Geometry: final body of the model. Coordinates: model frame, mm. A direction names the side the tool comes from. Give positions to 0.01 mm unless a question says otherwise; leave off trailing zeros. Order: outer loops, then holes, each group sorted by start corner. A loop starts at its lowest first (then second) coordinate and runs counter-clockwise, first axis right, second up. Notation, with made-up numbers: (8, 64) -> (52, 64) arc R22 cw to (52, 86) -> close; hole circle Ø7 at (34.5, 60.25). An arc over 180 degrees is marked (long way). One line per question, with ' | ' between items. Start each with the question number.
(1) Mould query, pull axis Z, two halves, no side actions, for faces 1 (the face through (1.4, -17.4, -40)), 2 (the face through (-7.66, 5.76, -1.7)), 3 (the face through (13.876, -6.451, -0.56)). Classes: +Z half, -Z half, draft (parallel to the pull), parting line (faces both ways), or undercut.
(2) First-contact query: pin 1 Ø3 at (y, z) = (-14, 29) entering from +X; pin 2 Ø4 at (y, z) = (5.68, 0) entering from -X; pin 3 Ø4 at (x, z) = (13.5, -26.5) entering from +Y. Flat tips, straight axial feed; report the tip coordinate or a pass-through.
(3) Section D-D (z = 0). State how many separate pieces and enclosed holes the cut face has, then the cut area to 3 significant figures.
(4) Set-up query: faces 4 (the face through (-10, 5, -2.85)), 5 (the face through (-13.907, -6.549, -0.56)), 6 (the face through (-10, 5, 4.856)). Return all of +Z, -Z, +X, -X, +Y, -Y with unobstructed straight access to the full face (end or side cutting, diameter ignored); none if empty.
(5) Section A-A (z = -13). Return loops of the section in (x, y), then the cut area to 3 significant figures.
(6) Section C-C (y = -13.5). Return loops of the section in (x, z).
(7) Section B-B (x = 0). Return loops of the section in (y, z), then the cut area to 3 significant figures.
(8) Ray query, L1, parallel to Y at x = -7.2, z = 0; L2, parallel to Y at x = -11.5, z = -14; L3, parallel to Z at x = -9.5, y = 8. Return the intervals inside material, ascending.
```python
from build123d import *

# Parameters (mm, degrees)
EXTRUDE_1_DEPTH     = 40
CUT_EXTRUDE_3_DEPTH = 81
SKETCH_8_R          = 6.65
CUT_EXTRUDE_4_DEPTH = 21
SKETCH_9_R          = 8.65
SKETCH_9_R_2        = 6.65
EXTRUDE_2_DEPTH     = 10
SKETCH_10_W         = 2.6
SKETCH_10_H         = 5.7
EXTRUDE_3_DEPTH     = 10
SKETCH_11_R         = 1.7
CUT_EXTRUDE_5_DEPTH = 10
FILLET_1_R          = 1


with BuildPart() as part:
    # 草图1 → 凸台-拉伸1 (new body, symmetric)
    with BuildSketch(Plane.XY):
        Polygon((-15, 0), (15, 0), (18.130448736, -10), (15, -20), (-15, -20), (-18.130448736, -10), align=None)
    extrude(amount=EXTRUDE_1_DEPTH, both=True)

    # 草图7 → 切除-拉伸3 (cut, through all)
    with BuildSketch(Plane(origin=(0, 0, -40), x_dir=(-1, 0, 0), z_dir=(0, 0, -1))):
        Polygon((14.986888042, -10), (12.795573927, -3), (-12.795573927, -3), (-14.986888042, -10), (-12.795573927, -17), (12.795573927, -17), align=None)
    extrude(amount=-CUT_EXTRUDE_3_DEPTH, mode=Mode.SUBTRACT)

    # 草图8 → 切除-拉伸4 (cut, through all)
    with BuildSketch(Plane(origin=(0, 0, 0), x_dir=(1, 0, 0), z_dir=(0, 1, 0))):
        Circle(SKETCH_8_R)
    extrude(amount=-CUT_EXTRUDE_4_DEPTH, mode=Mode.SUBTRACT)

    # 草图9 → 凸台-拉伸2 (add)
    with BuildSketch(Plane(origin=(0, 0, 0), x_dir=(1, 0, 0), z_dir=(0, 1, 0))):
        Circle(SKETCH_9_R)
        Circle(SKETCH_9_R_2, mode=Mode.SUBTRACT)
    extrude(amount=EXTRUDE_2_DEPTH)

    # 草图10 → 凸台-拉伸3 (add)
    with BuildSketch(Plane(origin=(0, 0, 0), x_dir=(1, 0, 0), z_dir=(0, 1, 0))):
        with BuildLine():
            ThreePointArc((-7.158670401, -4.855505955), (-8.65, 0), (-7.158670401, 4.855505955))
            Line((-7.158670401, 4.855505955), (-13.461589548, 4.855505955))
            Line((-13.461589548, 4.855505955), (-13.461589548, -4.855505955))
            Line((-13.461589548, -4.855505955), (-7.158670401, -4.855505955))
        make_face()
        with Locations((-10.161589548, 0)):
            Rectangle(SKETCH_10_W, SKETCH_10_H, mode=Mode.SUBTRACT)
    extrude(amount=EXTRUDE_3_DEPTH)

    # 草图11 → 切除-拉伸5 (cut)
    with BuildSketch(Plane.ZY.offset(13.461589548)):
        with Locations((0, 5.684678401)):
            Circle(SKETCH_11_R)
    extrude(amount=-CUT_EXTRUDE_5_DEPTH, mode=Mode.SUBTRACT)

    # 圆角1
    fillet_1_edges = [part.edges().sort_by_distance(p)[0] for p in [
        (-13.461589548, 5, -4.855505955),
        (-13.461589548, 5, 4.855505955),
        (-7.158670401, 5, 4.855505955),
        (-7.158670401, 5, -4.855505955),
    ]]
    fillet(fillet_1_edges, radius=FILLET_1_R)


solid = part.part
```
Response:
1) face 1: -Z half | face 2: undercut | face 3: draft
2) pin 1: stops at x = 17.35 | pin 2: stops at x = -13.46 | pin 3: stops at y = 0
3) separate pieces: 4 | enclosed holes: 0 | area: 242 mm^2
4) face 4: +Y | face 5: +Z, -Z | face 6: +Z, -X, +Y
5) outline: (-18.13, -10) -> (-15, -20) -> (15, -20) -> (18.13, -10) -> (15, 0) -> (-15, 0) -> close; hole (-14.99, -10) -> (-12.8, -17) -> (12.8, -17) -> (14.99, -10) -> (12.8, -3) -> (-12.8, -3) -> close | area: 274 mm^2
6) outline: (-17.03, -40) -> (-13.89, -40) -> (-13.89, 40) -> (-17.03, 40) -> close; (13.89, -40) -> (17.03, -40) -> (17.03, 40) -> (13.89, 40) -> close
7) outline: (-20, -40) -> (-17, -40) -> (-17, -6.65) -> (-20, -6.65) -> close; (-20, 6.65) -> (-17, 6.65) -> (-17, 40) -> (-20, 40) -> close; (-3, -40) -> (0, -40) -> (0, -8.65) -> (10, -8.65) -> (10, -6.65) -> (-3, -6.65) -> close; (-3, 6.65) -> (10, 6.65) -> (10, 8.65) -> (0, 8.65) -> (0, 40) -> (-3, 40) -> close | area: 440 mm^2
8) L1: y = -20 to -17, -3 to 3.98, 7.38 to 10 | L2: y = -20 to -17, -3 to 0 | L3: z = -4.86 to -2.85, 2.85 to 4.86
